Build history of the part. All positions in model axes, mm. A direction names the side the tool comes from. Round coordinates to 2 decimals unless told otherwise and drop trailing zeros. Write each loop counter-clockwise with the first axis right and the second up, starting at its lowest first coordinate (ties: lowest second). Pieces come first, ordered by that corner, then holes.
Autodesk Inventor part; units mm, degrees
ref_plane "YZ Plane" through (0, 0, 0) normal (1, 0, 0) x (0, 1, 0)
ref_plane "XZ Plane" through (0, 0, 0) normal (0, 1, 0) x (-1, 0, 0)
ref_plane "XY Plane" through (0, 0, 0) normal (0, 0, 1) x (1, 0, 0)
sketch "スケッチ1" plane through (0, 0, 0) normal (0, 1, 0) x (-1, 0, 0)
  line L0 (10.825, 21.65) -> (-10.825, 21.65)
  line L1 (-10.825, 21.65) -> (-10.825, -21.65)
  line L2 (-10.825, -21.65) -> (10.825, -21.65)
  line L3 (10.825, -21.65) -> (10.825, 21.65)
  line L4 (0, -42.6095) -> (0, 37.4005)
  line L5 (-15.3503, 0) -> (16.327, 0)
  point P0 (0, 0)
  dimension "d0" = 21.65
  dimension "d1" = 43.3
extrude "押し出し1" add sketch "スケッチ1" along normal blind 16
sketch "スケッチ2" plane through (0, 16, 0) normal (0, 1, 0) x (1, 0, 0)
  line L0 (-10.825, -28.575) -> (10.825, -28.575)
  line L1 (10.825, -28.575) -> (10.825, 28.575)
  line L2 (10.825, 28.575) -> (-10.825, 28.575)
  line L3 (-10.825, 28.575) -> (-10.825, -28.575)
  line L4 (15.155, 0) -> (-15.155, 0)
  point P0 (0, 0)
  point P1 (-10.825, -21.65)
  point P2 (10.825, -21.65)
  dimension "d4" = 57.15
extrude "押し出し2" add sketch "スケッチ2" along normal blind 5
sketch "スケッチ3" plane through (0, 21, 0) normal (0, 1, 0) x (1, 0, 0)
  circle A0 centre (-6, -25.5) radius 1.5
  circle A1 centre (6, -25.5) radius 1.5
  circle A2 centre (-6, 25.5) radius 1.5
  circle A3 centre (6, 25.5) radius 1.5
  line L0 (15.155, 0) -> (-15.155, 0)
  line L1 (0, 40.005) -> (0, -40.005)
  point P0 (0, 0)
  dimension "d9" = 3
  dimension "d10" = 3
  dimension "d11" = 3
  dimension "d12" = 3
  dimension "d13" = 12
  dimension "d14" = 12
  dimension "d15" = 51
  dimension "d16" = 51
extrude "押し出し3" cut sketch "スケッチ3" against normal up to next
sketch "スケッチ4" plane through (0, 21, 0) normal (0, 1, 0) x (1, 0, 0)
  line L0 (10.825, 21.65) -> (-10.825, 21.65)
  line L1 (-10.825, -21.65) -> (10.825, -21.65)
  line L2 (-10.825, 28.575) -> (-10.825, -28.575)
  line L3 (10.825, -28.575) -> (10.825, 28.575)
  point P0 (0, 0)
extrude "押し出し4" add sketch "スケッチ4" along normal blind 2
sketch "スケッチ5" plane through (0, 23, 0) normal (0, 1, 0) x (1, 0, 0)
  circle A0 centre (0, -11.5) radius 3
  circle A1 centre (6, -25.5) radius 1.5
  line L0 (0, 40.005) -> (0, -40.005)
  point P0 (0, 0)
  dimension "d21" = 14
  dimension "d22" = 6
extrude "押し出し5" add sketch "スケッチ5" along normal blind 3.6 contours A0 L0 | L0 A0
properties part number "servo"
1) Slice it at B-B (x = 6). Write the cut outline in (y, z) (3 decimals), plus the area to 3 significant figures.
Results:
outline: (0, -21.65) - (16, -21.65) - (16, -24) - (21, -24) - (21, -21.65) - (23, -21.65) - (23, 21.65) - (21, 21.65) - (21, 24) - (16, 24) - (16, 21.65) - (0, 21.65) - close; (16, -28.575) - (21, -28.575) - (21, -27) - (16, -27) - close; (16, 27) - (21, 27) - (21, 28.575) - (16, 28.575) - close
area: 1,040 mm2
2) Wall check: L1, parallel to X at y = 18.4, z = 25.5 (3 decimals); L2, parallel to Z at x = -6, y = 19.8 (3 decimals); L3, parallel to Y at x = -7, z = -1. Give the ranges that are in metal, low to high.
Results:
L1: x = -10.825 to -7.5, -4.5 to 4.5, 7.5 to 10.825
L2: z = -28.575 to -27, -24 to 24, 27 to 28.575
L3: y = 0 to 23
3) Which spindle directions (+Z, -Z, +X, -X, +Y, -Y) get a long thin tool onto all of the face, cutting with end or side? Do faces 5 (the flat face through (0, 16, 25)), 6 (the flat face through (0, 26.6, 11)), 7 (the flat face through (0, 16, -25)), 8 (the flat face through (0, 21, -25)), 9 (the flat face through (0, 22, 21.65)). Say none if no direction does.
Results:
face 5: +Z, +X, -X, -Y
face 6: +Z, -Z, +X, -X, +Y
face 7: -Z, +X, -X, -Y
face 8: -Z, +X, -X, +Y
face 9: +Z, +X, -X, +Y
4) Slice it at D-D (x = 0). Write the cut outline in (y, z) (3 decimals).
Results:
outline: (0, -21.65) - (16, -21.65) - (16, -28.575) - (21, -28.575) - (21, -21.65) - (23, -21.65) - (23, 8.5) - (26.6, 8.5) - (26.6, 14.5) - (23, 14.5) - (23, 21.65) - (21, 21.65) - (21, 28.575) - (16, 28.575) - (16, 21.65) - (0, 21.65) - close
5) Slice it at C-C (y = 18.25). Write the cut outline in (x, z) (3 decimals), plus the area to 3 significant figures.
Results:
outline: (-10.825, -28.575) - (10.825, -28.575) - (10.825, 28.575) - (-10.825, 28.575) - close; hole circle Ø3 at (-6, -25.5); hole circle Ø3 at (-6, 25.5); hole circle Ø3 at (6, -25.5); hole circle Ø3 at (6, 25.5)
area: 1,210 mm2
6) Slice it at A-A (z = -25.5). Write the cut outline in (x, y) (3 decimals), plus the area to 4 significant figures.
Results:
outline: (-10.825, 16) - (-7.5, 16) - (-7.5, 21) - (-10.825, 21) - close; (-4.5, 16) - (4.5, 16) - (4.5, 21) - (-4.5, 21) - close; (7.5, 16) - (10.825, 16) - (10.825, 21) - (7.5, 21) - close
area: 78.25 mm2
7) Mould opens along X. For faces 1 (the cylindrical face through (6, 19, 24)), 2 (the cylindrical face through (-6, 19, -27)), 3 (the cylindrical face through (-0.65, 24.77, 8.57)), 4 (the flat face through (0, 8, -21.65)) say: released by +X, released by -X, zero draft, split by the parting line, or undercut.
Results:
face 1: undercut
face 2: undercut
face 3: split by the parting line
face 4: zero draft
8) Pin check, flat tips, straight feed: pin 1 Ø5 at (x, y) = (5, 5) entering from +Z; pin 2 Ø2 at (x, z) = (-3, -26.5) entering from -Y; pin 3 Ø1.6 at (x, y) = (1, 22.5) entering from -Z; pin 4 Ø2.5 at (x, z) = (6, -25.5) entering from -Y. Stop position of each tip, or through.
Results:
pin 1: stops at z = 21.65
pin 2: stops at y = 16
pin 3: stops at z = -21.65
pin 4: passes through
